Verification items for the finished model (mm, model axes). A direction names the side the tool comes from. Give positions to 0.01 mm unless a question says otherwise; leave off trailing zeros. Loops run counter-clockwise (first coordinate to the right, second up) from the corner with the lowest first, then second, coordinate; pieces in that order, holes last. Notation, with made-up numbers: M -29,-36 L 20,-36 A18 cw 20,-7 Z; hole C 15,-17 d1. An arc over 180 degrees is marked long. Answer in a Markdown table with one row per item.
```python
from build123d import *

# Parameters (mm, degrees)
BASE_FLANGE1_DEPTH = 3.175
SKETCH6_R          = 3.3782
CUT_EXTRUDE1_DEPTH = 251.203228354
SKETCH7_R          = 3.3782
CUT_EXTRUDE2_DEPTH = 251.203228354


# Sheet-metal steps are written as plain solids
with BuildPart() as part:
    # Sketch1 → Base-Flange1 (new body)
    with BuildSketch(Plane.XY):
        with BuildLine():
            Line((37.764632708, 0), (182.767027516, 0))
            ThreePointArc((182.767027516, 0), (199.281906874, 9.554671686), (199.230460753, 28.63425094))
            Line((199.230460753, 28.63425094), (135.335454487, 138.390472515))
            ThreePointArc((135.335454487, 138.390472515), (119.911781029, 147.827825072), (103.551346546, 140.127856906))
            Line((103.551346546, 140.127856906), (22.443958003, 30.371635332))
            ThreePointArc((22.443958003, 30.371635332), (20.756110534, 10.470217167), (37.764632708, 0))
        make_face()
    extrude(amount=-BASE_FLANGE1_DEPTH)

    # Sketch6 → Cut-Extrude1 (cut, through all)
    with BuildSketch(Plane.XY):
        with Locations((52.14616343, 35.306)):
            Circle(SKETCH6_R)
        with BuildLine():
            ThreePointArc((119.02436343, 35.306), (111.857415274, 65.4267576), (91.892651201, 89.091781998))
            ThreePointArc((91.892651201, 89.091781998), (87.168081554, 88.382619016), (87.877244536, 83.658049369))
            ThreePointArc((87.877244536, 83.658049369), (105.82505941, 62.383794622), (112.26796343, 35.306))
            ThreePointArc((112.26796343, 35.306), (115.64616343, 31.9278), (119.02436343, 35.306))
        make_face()
    extrude(amount=-CUT_EXTRUDE1_DEPTH, mode=Mode.SUBTRACT)

    # Sketch7 → Cut-Extrude2 (cut, through all)
    with BuildSketch(Plane.XY):
        with Locations((57.037027516, 12.7)):
            Circle(SKETCH7_R)
        with Locations((189.117027516, 12.7)):
            Circle(SKETCH7_R)
    extrude(amount=-CUT_EXTRUDE2_DEPTH, mode=Mode.SUBTRACT)


solid = part.part
```
Item 1: Sectioned sample at B-B (y = 12.7). Record the cut outline in (x, z) (3 decimals).
Reported:
| item | result |
|---|---|
| outline | M 19.804,-3.175 L 53.659,-3.175 L 53.659,0 L 19.804,0 Z; M 60.415,-3.175 L 185.739,-3.175 L 185.739,0 L 60.415,0 Z; M 192.495,-3.175 L 200.728,-3.175 L 200.728,0 L 192.495,0 Z |
Item 2: Sectioned sample at C-C (y = 108). Record the cut outline in (x, z) (3 decimals).
Reported:
| item | result |
|---|---|
| outline | M 79.81,-3.175 L 153.027,-3.175 L 153.027,0 L 79.81,0 Z |
Item 3: Release check for a two-part mould opening along Y. For faces 3 (the cylindrical face through (60.26, 13.71, -1.57)), 4 (the cylindrical face through (120.18, 147.81, -1.57)), 5 (the flat face through (109, 42, -3.175)) record: released by +Y, released by -Y, zero draft, split by the parting line, or undercut.
Reported:
| item | result |
|---|---|
| face 3 | undercut |
| face 4 | released by +Y |
| face 5 | zero draft |
Item 4: Sectioned sample at A-A (z = -2.6). Record the cut outline in (x, y).
Reported:
| item | result |
|---|---|
| outline | M 22.44,30.37 A19.05 ccw 37.76,0 L 182.77,0 A19.05 ccw 199.23,28.63 L 135.34,138.39 A19.05 ccw 103.55,140.13 Z; hole C 52.15,35.31 d6.76; hole C 57.04,12.7 d6.76; hole M 87.88,83.66 A60.12 cw 112.27,35.31 A3.38 ccw 119.02,35.31 A66.88 ccw 91.89,89.09 A3.38 ccw Z; hole C 189.12,12.7 d6.76 |
Item 5: Tool access check on faces 1 (the cylindrical face through (105.65, 62.73, -1.57)), 2 (the cylindrical face through (20.626, 10.734, -1.565)). Record the directions out of +Z, -Z, +X, -X, +Y, -Y that give a thin tool (end or side, any length) a straight path to the whole face; none if there is none.
Reported:
| item | result |
|---|---|
| face 1 | +Z, -Z |
| face 2 | +Z, -Z, -X |
Item 6: Go/stop test with flat-tipped pins: pin 1 (4 mm diameter, centred on x = 52.15, y = 35.31, fed in from +Z) (1 decimal); pin 2 (1.5 mm diameter, centred on y = 65, z = -1.5, fed in from +X). Record where each tip stops, or that it passes through.
Reported:
| item | result |
|---|---|
| pin 1 | passes through |
| pin 2 | stops at x = 178.5 |
Item 7: Sectioned sample at D-D (x = 66). Record the cut outline in (y, z) (3 decimals).
Reported:
| item | result |
|---|---|
| outline | M 0,-3.175 L 89.313,-3.175 L 89.313,0 L 0,0 Z |
Item 8: Scan lines: L1, parallel to X at y = 60.5, z = -2.85; L2, parallel to X at y = 45, z = -0.4; L3, parallel to Y at x = 179.5, z = -2.55. Record each from-to range of solid material in increasing order. Write a range as [from, to].
Reported:
| item | result |
|---|---|
| L1 | x = [44.71, 106.73], [114.1, 180.68] |
| L2 | x = [33.25, 111.48], [118.32, 189.7] |
| L3 | y = [0, 62.53] |
